Part model, mm, in its own coordinate system. Face numbers are marked on the shaded views. A direction names the side the tool comes from. Round coordinates to 2 decimals unless told otherwise and drop trailing zeros. Loops run counter-clockwise (first coordinate to the right, second up) from the corner with the lowest first, then second, coordinate; pieces in that order, holes last. Notation, with made-up numbers: M -2.5,50.5 L 33.5,50.5 A12 ccw 33.5,59.5 Z; hole C 55.25,-37 d11. An arc over 180 degrees is marked long. Put each result on its own line as item: value. Start each with the question number.
1) Pull direction Z, two halves, no side cores. Call the marked faces 3, 4 and 5: +Z half, -Z half, draft (parallel to the pull), parting line (faces both ways), or undercut.
2) Slice it at D-D on z = -4. Give the cut face in (x, y), then the cut area to 3 significant figures.
3) Drop flat-ended pins along their axis: pin 1 Ø5.5 at (x, z) = (-5, 0) entering from -Y; pin 2 Ø4 at (y, z) = (4.5, 3.5) entering from -X. Give the stop position or say it passes through.
4) Which spindle directions (+Z, -Z, +X, -X, +Y, -Y) get a long thin tool onto all of the face, cutting with end or side? Do the marked faces 1 and 2. Say none if no direction does.
5) Probe line 1 along Y through (x, z) = (12.8, 0); line 2 along Y through (x, z) = (1.75, -2.5); line 3 along X through (y, z) = (6, 0.75). List the from-to ranges inside material, lowest first.
6) Slice it at C-C on y = 2. Give the cut face in (x, z).
7) Slice it at B-B on z = 0. Give the cut face in (x, y), then the cut area to 3 significant figures.
8) Slice it at A-A on x = -5. Give the cut face in (y, z).
```python
from build123d import *

# Parameters (mm, degrees)
SKETCH1_W                          = 30
SKETCH1_H                          = 23
BOSS_EXTRUDE1_DEPTH                = 5
SKETCH2_W                          = 26
SKETCH2_H                          = 19
CUT_EXTRUDE1_DEPTH                 = 22.38340478
CHAMFER1_SIZE                      = 1.5
TAPPED_HOLE_FOR_M4X0_7_HELICOIL1_D = 4.2
M3_CLEARANCE_HOLE1_D               = 3.2
M3_TAPPED_HOLE1_D                  = 2.5


with BuildPart() as part:
    # Sketch1 → Boss-Extrude1 (new, symmetric)
    with BuildSketch(Plane.XY):
        Rectangle(SKETCH1_W, SKETCH1_H)
    extrude(amount=BOSS_EXTRUDE1_DEPTH, both=True)

    # Sketch2 → Cut-Extrude1 (cut, through all)
    with BuildSketch(Plane.XY.offset(5)):
        with Locations((-2, -2)):
            Rectangle(SKETCH2_W, SKETCH2_H)
    extrude(amount=-CUT_EXTRUDE1_DEPTH, mode=Mode.SUBTRACT)

    # Chamfer1
    chamfer1_edges = [part.edges().sort_by_distance(p)[0] for p in [
        (15, 11.5, 0),
    ]]
    chamfer(chamfer1_edges, length=CHAMFER1_SIZE)

    # Tapped Hole for M4x0.7 Helicoil1 (through all)
    with Locations(Plane(origin=(0, 11.5, 0), x_dir=(1, 0, 0), z_dir=(0, 1, 0))):
        with Locations((-5, 0)):
            Hole(TAPPED_HOLE_FOR_M4X0_7_HELICOIL1_D / 2)

    # M3 Clearance Hole1 (through all)
    with Locations(Plane(origin=(15, 0, 0), x_dir=(0, 0, -1), z_dir=(1, 0, 0))):
        with Locations((0, -8.232), (0, 3.198)):
            Hole(M3_CLEARANCE_HOLE1_D / 2)

    # M3 Tapped Hole1 (through all)
    with Locations(Plane(origin=(15, 0, 0), x_dir=(0, 0, -1), z_dir=(1, 0, 0))):
        with Locations((0, -2.517)):
            Hole(M3_TAPPED_HOLE1_D / 2)


solid = part.part
```
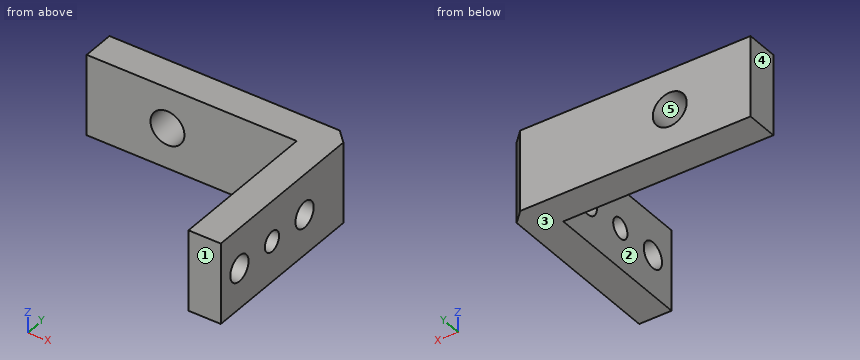
Recorded:
1. face 3: -Z half
1. face 4: draft
1. face 5: undercut
2. outline: M -15,7.5 L 11,7.5 L 11,-11.5 L 15,-11.5 L 15,10 L 13.5,11.5 L -15,11.5 Z
2. area: 195 mm2
3. pin 1: stops at y = 7.5
3. pin 2: stops at x = 11
4. face 1: +Z, -Z, +X, -X, -Y
4. face 2: +Z, -Z, -X, -Y
5. line 1: y = -11.5 to -9.83, -6.63 to -3.77, -1.27 to 1.6, 4.8 to 11.5
5. line 2: y = 7.5 to 11.5
5. line 3: x = 11 to 15
6. outline: M 11,-5 L 15,-5 L 15,-1.06 L 11,-1.06 Z; M 11,1.06 L 15,1.06 L 15,5 L 11,5 Z
7. outline: M -15,7.5 L -7.1,7.5 L -7.1,11.5 L -15,11.5 Z; M -2.9,7.5 L 11,7.5 L 11,4.8 L 15,4.8 L 15,10 L 13.5,11.5 L -2.9,11.5 Z; M 11,-11.5 L 15,-11.5 L 15,-9.83 L 11,-9.83 Z; M 11,-6.63 L 15,-6.63 L 15,-3.77 L 11,-3.77 Z; M 11,-1.27 L 15,-1.27 L 15,1.6 L 11,1.6 Z
7. area: 142 mm2
8. outline: M 7.5,-5 L 11.5,-5 L 11.5,-2.1 L 7.5,-2.1 Z; M 7.5,2.1 L 11.5,2.1 L 11.5,5 L 7.5,5 Z
